from build123d import *

# Parameters (mm, degrees)
SKETCH1_R               = 30
BOSS_EXTRUDE1_DEPTH     = 14
SKETCH2_R               = 11.05
CUT_EXTRUDE1_DEPTH      = 15
SKETCH5_W               = 8
SKETCH5_H               = 40
BOSS_EXTRUDE2_DEPTH     = 80
FILLET1_R               = 10
SKETCH12_R              = 11
CUT_EXTRUDE5_DEPTH      = 15.5
CUT_EXTRUDE5_DEPTH_BACK = 15.5
SKETCH13_R              = 5.75
CUT_EXTRUDE6_DEPTH      = 33
SKETCH14_W              = 5
SKETCH14_H              = 60.1
CUT_EXTRUDE7_DEPTH      = 5
FILLET2_R               = 1
FILLET3_R               = 1
SKETCH15_W              = 4
SKETCH15_H              = 5
CUT_EXTRUDE14_DEPTH     = 33


with BuildPart() as part:
    # Sketch1 → Boss-Extrude1 (new body)
    with BuildSketch(Plane(origin=(0, 0, 0), x_dir=(1, 0, 0), z_dir=(0, 1, 0))):
        Circle(SKETCH1_R)
    extrude(amount=BOSS_EXTRUDE1_DEPTH)

    # Sketch2 → Cut-Extrude1 (cut, through all)
    with BuildSketch(Plane.XZ):
        Circle(SKETCH2_R)
    extrude(amount=-CUT_EXTRUDE1_DEPTH, mode=Mode.SUBTRACT)

    # Sketch5 → Boss-Extrude2 (add)
    with BuildSketch(Plane(origin=(0, 14, 0), x_dir=(1, 0, 0), z_dir=(0, 1, 0))):
        with Locations((-12.5, 0)):
            Rectangle(SKETCH5_W, SKETCH5_H)
        with Locations((12.5, 0)):
            Rectangle(SKETCH5_W, SKETCH5_H)
    extrude(amount=BOSS_EXTRUDE2_DEPTH)

    # Fillet1
    fillet1_edges = [part.edges().sort_by_distance(p)[0] for p in [
        (-12.5, 94, 20),
        (-12.5, 94, -20),
        (12.5, 94, 20),
        (12.5, 94, -20),
    ]]
    fillet(fillet1_edges, radius=FILLET1_R)

    # Sketch12 → Cut-Extrude5 (cut, two sides)
    with BuildSketch(Plane(origin=(0, 0, 0), x_dir=(0, 0, -1), z_dir=(1, 0, 0))) as cut_extrude5_sk:
        with Locations((0, 79)):
            Circle(SKETCH12_R)
    extrude(amount=CUT_EXTRUDE5_DEPTH, mode=Mode.SUBTRACT)
    extrude(cut_extrude5_sk.sketch, amount=-CUT_EXTRUDE5_DEPTH_BACK, mode=Mode.SUBTRACT)

    # Sketch13 → Cut-Extrude6 (cut)
    with BuildSketch(Plane.ZY.offset(16.5)):
        with Locations((0, 79)):
            Circle(SKETCH13_R)
    extrude(amount=-CUT_EXTRUDE6_DEPTH, mode=Mode.SUBTRACT)

    # Sketch14 → Cut-Extrude7 (cut)
    with BuildSketch(Plane(origin=(0, 14, 0), x_dir=(1, 0, 0), z_dir=(0, 1, 0))):
        with Locations((-20, 0)):
            Rectangle(SKETCH14_W, SKETCH14_H)
        with Locations((20, 0)):
            Rectangle(SKETCH14_W, SKETCH14_H)
    extrude(amount=-CUT_EXTRUDE7_DEPTH, mode=Mode.SUBTRACT)

    # Fillet2
    fillet2_edges = [part.edges().sort_by_distance(p)[0] for p in [
        (-16.5, 94, 0),
        (-16.5, 49, 20),
        (-16.5, 49, -20),
        (-16.5, 91.071067812, 17.071067812),
        (-16.5, 91.071067812, -17.071067812),
        (16.5, 94, 0),
        (16.5, 49, -20),
        (16.5, 49, 20),
        (16.5, 91.071067812, 17.071067812),
        (16.5, 91.071067812, -17.071067812),
    ]]
    fillet(fillet2_edges, radius=FILLET2_R)

    # Fillet3
    fillet3_edges = [part.edges().sort_by_distance(p)[0] for p in [
        (-8.5, 94, 0),
        (-8.5, 49, -20),
        (-8.5, 49, 20),
        (-8.5, 91.071067812, 17.071067812),
        (-8.5, 91.071067812, -17.071067812),
        (8.5, 94, 0),
        (8.5, 49, 20),
        (8.5, 49, -20),
        (8.5, 91.071067812, 17.071067812),
        (8.5, 91.071067812, -17.071067812),
    ]]
    fillet(fillet3_edges, radius=FILLET3_R)

    # Sketch15 → Cut-Extrude14 (cut)
    with BuildSketch(Plane(origin=(16.5, 0, 0), x_dir=(0, 0, -1), z_dir=(1, 0, 0))):
        with Locations((-14, 79)):
            Rectangle(SKETCH15_W, SKETCH15_H)
    extrude(amount=-CUT_EXTRUDE14_DEPTH, mode=Mode.SUBTRACT)


solid = part.part
Source: CAD feature listing. Evaluate the final solid. Frame: model axes, mm. A direction names the side the tool comes from. Coordinates: 2 decimals unless noted, no trailing zeros. Loops run counter-clockwise (first coordinate to the right, second up) from the corner with the lowest first, then second, coordinate; pieces in that order, holes last. Notation, with made-up numbers: (73.25, 38) -> (117.25, 38) arc R25 ccw to (117.25, 55) -> close; hole circle Ø11 at (-7.5, -7.5). An arc over 180 degrees is marked (long way). Answer in a Markdown table with one row per item. Add a question column.
Q1. Section D-D on z = -22. Return the cut outline in (x, y), and give its area (3 significant figures).
Q2. Contact query for flat-ended pins moving along their axis: pin 1 Ø10 at (x, y) = (-14, 55) entering from +Z; pin 2 Ø2 at (x, z) = (-11.5, -4.5) entering from -Y; pin 3 Ø5 at (x, y) = (16.5, 75.5) entering from -Z; pin 4 Ø10.5 at (x, z) = (-2, -7.5) entering from +Y. Output: stop coordinate, or through.
Q3. Reachability of faces 1 (the face through (13, 81.5, 14)), 2 (the face through (11.951, 89.906, 1.432)), 3 (the face through (-13, 49, -20)), 4 (the face through (-16.5, 53, 0)) from +Z, -Z, +X, -X, +Y, -Y: full face, straight path, thin tool, end or side. Return the list, or none.
Q4. Section A-A on x = 0. Return the cut outline in (y, z), and give its area (3 significant figures).
Q5. Section C-C on y = 79. Give the number of separate pieces and of enclosed holes in the cut face, and give its area (3 significant figures).
Q6. Ray query, line 1 along Y through (x, z) = (14, 0); line 2 along X through (y, z) = (66, 10); line 3 along Z through (x, y) = (12.25, 79). Return the intervals inside material, ascending.
Q7. Section B-B on y = 46.5. Return the cut outline in (x, z).
Q8. Pull-direction query (X, two-part tool) for faces 5 (the face through (-22.5, 12, 0)), 6 (the face through (13, 79, 12)), 7 (the face through (16.5, 53, 0)); classes: pulls with the +X half, pulls with the -X half, needs draft (parallel to the pull), parting line crosses it, or undercut.
Computed values:
| question | item | result |
|---|---|---|
| 1 | outline | (-20.4, 0) -> (20.4, 0) -> (20.4, 9) -> (17.5, 9) -> (17.5, 14) -> (-17.5, 14) -> (-17.5, 9) -> (-20.4, 9) -> close |
| 1 | area | 542 mm^2 |
| 2 | pin 1 | stops at z = 20 |
| 2 | pin 2 | stops at y = 0 |
| 2 | pin 3 | stops at z = -20 |
| 2 | pin 4 | stops at y = 14 |
| 3 | face 1 | +X, -X |
| 3 | face 2 | none |
| 3 | face 3 | -Z, +X, -X, +Y |
| 3 | face 4 | +Z, -Z, -X, +Y |
| 4 | outline | (0, -30) -> (14, -30) -> (14, -11.05) -> (0, -11.05) -> close; (0, 11.05) -> (14, 11.05) -> (14, 30) -> (0, 30) -> close |
| 4 | area | 531 mm^2 |
| 5 | separate pieces | 6 |
| 5 | enclosed holes | 0 |
| 5 | area | 243 mm^2 |
| 6 | line 1 | y = 0 to 68, 90 to 94 |
| 6 | line 2 | x = -16.5 to -8.5, 8.5 to 16.5 |
| 6 | line 3 | z = -20 to -11, 11 to 12, 16 to 20 |
| 7 | outline | (-16.5, -19) arc R1 ccw to (-15.5, -20) -> (-9.5, -20) arc R1 ccw to (-8.5, -19) -> (-8.5, 19) arc R1 ccw to (-9.5, 20) -> (-15.5, 20) arc R1 ccw to (-16.5, 19) -> close; (8.5, -19) arc R1 ccw to (9.5, -20) -> (15.5, -20) arc R1 ccw to (16.5, -19) -> (16.5, 19) arc R1 ccw to (15.5, 20) -> (9.5, 20) arc R1 ccw to (8.5, 19) -> close |
| 8 | face 5 | undercut |
| 8 | face 6 | needs draft |
| 8 | face 7 | pulls with the +X half |
